Can you work these out from the model? Positions are in its coordinate system, mm. Round coordinates to 2 decimals unless told otherwise and drop trailing zeros. Order: outer loops, then holes, each group sorted by start corner. A loop starts at its lowest first (then second) coordinate and runs counter-clockwise, first axis right, second up. Notation, with made-up numbers: (44.25, 9) - (53.25, 9) arc R23 cw to (53.25, 20) - close; hole circle Ø2 at (-28, 59). An arc over 180 degrees is marked (long way). Write item = value, one per line.
Autodesk Inventor part; units mm, degrees
ref_plane "YZ Plane" through (0, 0, 0) normal (1, 0, 0) x (0, 1, 0)
ref_plane "XZ Plane" through (0, 0, 0) normal (0, 1, 0) x (-1, 0, 0)
ref_plane "XY Plane" through (0, 0, 0) normal (0, 0, 1) x (1, 0, 0)
sketch "スケッチ1" plane through (0, 0, 0) normal (0, 0, 1) x (1, 0, 0)
  circle A0 centre (0, 0) radius 10
  circle A1 centre (0, 0) radius 50 construction
  circle A2 centre (0, -28) radius 11.9375 construction
  circle A3 centre (-0.2119, 34.8748) radius 11.9375 construction
  circle A4 centre (0, -28) radius 15.9375 construction
  circle A5 centre (0, 0) radius 4 construction
  circle A6 centre (0, -28) radius 22.5 construction
  circle A7 centre (0, 300) radius 5 construction
  circle A8 centre (0, 300) radius 47.7465 construction
  line L0 (47.4611, 294.7873) -> (11.8661, -29.3033) construction
  line L1 (-47.4611, 294.7873) -> (-11.8661, -29.3033) construction
  circle A9 centre (-0.2119, 34.8748) radius 19.25 construction
  line L2 (-12.0776, 316.763) -> (11.6547, 316.763) construction
  line L3 (-22.6185, -92.0395) -> (22.1946, -92.0395) construction
  line L4 (22.5, -18) -> (-22.5, -18) construction
  line L5 (-22.5, -18) -> (-22.5, -38) construction
  line L6 (-22.5, -38) -> (22.5, -38) construction
  line L7 (22.5, -38) -> (22.5, -18) construction
  line L8 (22.5, -18) -> (-22.5, -38) construction
  line L9 (-22.5, -18) -> (22.5, -38) construction
  circle A10 centre (-22.5, -18) radius 1.6
  circle A11 centre (22.5, -18) radius 1.6
  circle A12 centre (22.5, -38) radius 1.6
  circle A13 centre (-22.5, -38) radius 1.6
  line L10 (30, 30) -> (-30, 30) construction
  line L11 (-30, 30) -> (-30, -30) construction
  line L12 (-30, -30) -> (30, -30) construction
  line L13 (30, -30) -> (30, 30) construction
  line L14 (30, 30) -> (-30, -30) construction
  line L15 (-30, 30) -> (30, -30) construction
  circle A14 centre (-30, 30) radius 1.25
  circle A15 centre (30, 30) radius 1.25
  circle A16 centre (30, -30) radius 1.25
  circle A17 centre (-30, -30) radius 1.25
  circle A18 centre (0, -28) radius 10
  circle A19 centre (0, 300) radius 1.75
  arc A20 (35, 30) -> (34.9923, 30.2769) centre (30, 30) ccw
  arc A21 (33.6477, -33.4197) -> (35, -30) centre (30, -30) ccw
  arc A22 (22.5, -43) -> (26.1477, -41.4197) centre (22.5, -38) ccw
  arc A23 (-26.1477, -41.4197) -> (-22.5, -43) centre (-22.5, -38) ccw
  arc A24 (-35, -30) -> (-33.6477, -33.4197) centre (-30, -30) ccw
  arc A25 (-34.9923, 30.2769) -> (-35, 30) centre (-30, 30) ccw
  arc A26 (19.9693, 301.1077) -> (-19.9693, 301.1077) centre (0, 300) ccw
  line L16 (-19.9693, 301.1077) -> (-34.9923, 30.2769)
  line L17 (-33.6477, -33.4197) -> (-26.1477, -41.4197)
  line L18 (19.9693, 301.1077) -> (34.9923, 30.2769)
  line L19 (33.6477, -33.4197) -> (26.1477, -41.4197)
  line L20 (22.5, -43) -> (-22.5, -43)
  circle A27 centre (-30, 0) radius 1.25
  circle A28 centre (30, 0) radius 1.25
  line L21 (-35, 30) -> (-35, -30)
  line L22 (35, -30) -> (35, 30)
  circle A29 centre (-30, 15) radius 1.6
  circle A30 centre (30, 15) radius 1.6
  circle A31 centre (-18, 242.7636) radius 1.6
  circle A32 centre (18, 242.7636) radius 1.6
  circle A33 centre (0, 300) radius 60 construction
  point P0 (0, 0)
  dimension "d0" = 20
  dimension "d1" = 100
  dimension "d11" = 23.875
  dimension "d12" = 23.875
  dimension "d16" = 8
  dimension "d17" = 45
  dimension "d18" = 28
  dimension "d19" = 4
  dimension "d26" = 10
  dimension "d27" = 300
  dimension "d28" = 95.493
  dimension "d30" = 38.5
  dimension "d36" = 45
  dimension "d37" = 20
  dimension "d38" = 3.2
  dimension "d39" = 3.2
  dimension "d40" = 3.2
  dimension "d41" = 3.2
  dimension "d46" = 60
  dimension "d47" = 60
  dimension "d48" = 2.5
  dimension "d49" = 2.5
  dimension "d50" = 2.5
  dimension "d51" = 2.5
  dimension "d52" = 20
  dimension "d53" = 3.5
  dimension "d55" = 5
  dimension "d56" = 5
  dimension "d57" = 20
  dimension "d58" = 5
  dimension "d59" = 5
  dimension "d60" = 5
  dimension "d61" = 5
  dimension "d64" = 2.5
  dimension "d65" = 2.5
  dimension "d66" = 3.2
  dimension "d67" = 3.2
  dimension "d68" = 15
  dimension "d69" = 3.2
  dimension "d70" = 3.2
  dimension "d71" = 120
  dimension "d72" = 36
extrude "押し出し2" add sketch "スケッチ1" along normal blind 4
properties part number "関節3_側板1" material "アルミニウム 6061"
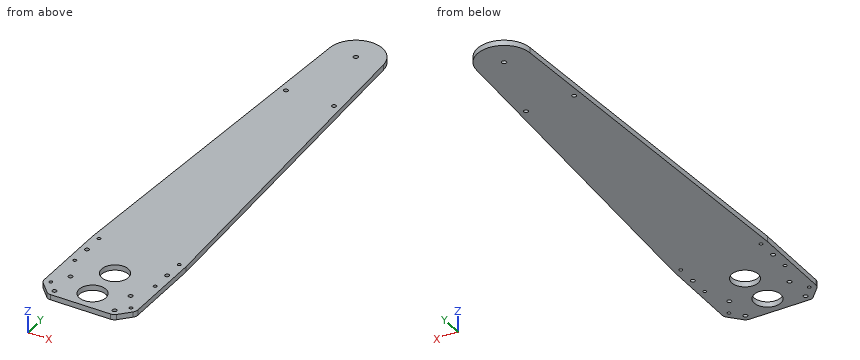
(1) If we section it at A-A (x = 7): Write out the boundary of the cut face in (y, z) (3 decimals).
Computed:
outline = (-43, 0) - (-35.141, 0) - (-35.141, 4) - (-43, 4) - close; (-20.859, 0) - (-7.141, 0) - (-7.141, 4) - (-20.859, 4) - close; (7.141, 0) - (318.735, 0) - (318.735, 4) - (7.141, 4) - close
(2) If we section it at C-C (y = 292.5): Write out the boundary of the cut face in (x, z), plus the area to 3 significant figures.
Computed:
outline = (-20.45, 0) - (20.45, 0) - (20.45, 4) - (-20.45, 4) - close
area = 164 mm^2
(3) Will this pin go through, and if not, where does the flat tip stop? P1, Ø1.5, axis at y = 101, z = 0.5, coming from the +X side.
Computed:
P1 = 31.11
(4) If we section it at D-D (y = 153.5): Write out the boundary of the cut face in (x, z), plus the area to 3 significant figures.
Computed:
outline = (-28.16, 0) - (28.16, 0) - (28.16, 4) - (-28.16, 4) - close
area = 225 mm^2
(5) If we section it at B-B (z = 2.4): State how many separate pieces and enclosed holes the cut face has, plus the area to 3 significant figures.
Computed:
separate_pieces = 1
enclosed_holes = 17
area = 19,800 mm^2
(6) If I drill on line 1 (X direction, y = 5.5, z = 1.3); line 2 (X direction, y = 225.5, z = 2); line 3 (X direction, y = 255.5, z = 3.75), over which ranges is the centre line in solid material (lowest first)? Write a range as from..to.
Computed:
line_1 = -35..-8.35, 8.35..35
line_2 = -24.16..24.16
line_3 = -22.5..22.5
